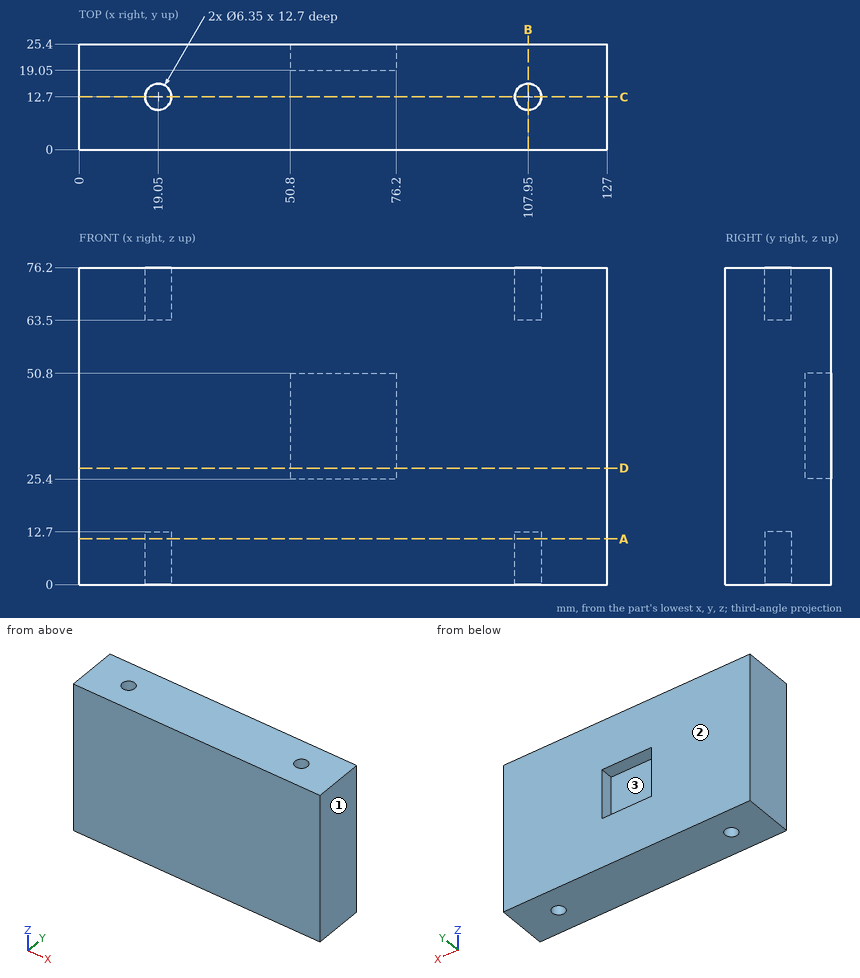
Geometry: see drawing. Coordinates: mm, zero at the bounding-box minimum. Coordinates: 2 decimals unless noted, no trailing zeros. Order: outer loops, then holes, each group sorted by start corner. A loop starts at its lowest first (then second) coordinate and runs counter-clockwise, first axis right, second up. Notation, with made-up numbers: (22.25, 21) - (51.25, 21) arc R14 ccw to (51.25, 47) - close; hole circle Ø8 at (-20.5, 17.5). An arc over 180 degrees is marked (long way). Return JSON: item names as keys, results as strings.
Q1. Cut plane D-D (z = 28). Return loops of the section in (x, y), then the cut area to 3 significant figures.
The answers:
{"outline": "(0, 0) - (127, 0) - (127, 25.4) - (76.2, 25.4) - (76.2, 19.05) - (50.8, 19.05) - (50.8, 25.4) - (0, 25.4) - close", "area": "3,060 mm2"}
Q2. Cut plane C-C (y = 12.7). Return loops of the section in (x, z) (3 decimals).
The answers:
{"outline": "(0, 0) - (15.875, 0) - (15.875, 12.7) - (22.225, 12.7) - (22.225, 0) - (104.775, 0) - (104.775, 12.7) - (111.125, 12.7) - (111.125, 0) - (127, 0) - (127, 76.2) - (111.125, 76.2) - (111.125, 63.5) - (104.775, 63.5) - (104.775, 76.2) - (22.225, 76.2) - (22.225, 63.5) - (15.875, 63.5) - (15.875, 76.2) - (0, 76.2) - close"}
Q3. First-contact query: pin 1 (12.5 mm diameter, centred on x = 68, z = 43, fed in from +Y); pin 2 (5.5 mm diameter, centred on x = 107.95, y = 12.7, fed in from +Z). Flat tips, straight axial feed; report the tip coordinate or a pass-through.
The answers:
{"pin 1": "stops at y = 19.05", "pin 2": "stops at z = 63.5"}
Q4. Ray query, probe 1 along Z at (x, y) = (66.5, 22.5); probe 2 along Y at (x, z) = (19.05, 7) (3 decimals); probe 3 along X at (y, z) = (22, 34.5). Return the intervals inside material, ascending.
The answers:
{"probe 1": "z = 0 to 25.4, 50.8 to 76.2", "probe 2": "y = 0 to 9.525, 15.875 to 25.4", "probe 3": "x = 0 to 50.8, 76.2 to 127"}
Q5. Draft query along X for the marked faces 1, 2 and 3. Return one class per face: +X half, -X half, draft (parallel to the pull), parting line (faces both ways), or undercut.
The answers:
{"face 1": "+X half", "face 2": "draft", "face 3": "undercut"}
Q6. Cut plane A-A (z = 11). Return loops of the section in (x, y) (3 decimals), then the cut area to 3 significant figures.
The answers:
{"outline": "(0, 0) - (127, 0) - (127, 25.4) - (0, 25.4) - close; hole circle Ø6.35 at (19.05, 12.7); hole circle Ø6.35 at (107.95, 12.7)", "area": "3,160 mm2"}
Q7. Cut plane B-B (x = 107.95). Return loops of the section in (y, z) (3 decimals).
The answers:
{"outline": "(0, 0) - (9.525, 0) - (9.525, 12.7) - (15.875, 12.7) - (15.875, 0) - (25.4, 0) - (25.4, 76.2) - (15.875, 76.2) - (15.875, 63.5) - (9.525, 63.5) - (9.525, 76.2) - (0, 76.2) - close"}
